Geometry check sheet. Reference: the model listing, model coordinates, mm. Round coordinates to 2 decimals unless told otherwise and drop trailing zeros. Order: outer loops, then holes, each group sorted by start corner. A loop starts at its lowest first (then second) coordinate and runs counter-clockwise, first axis right, second up. Notation, with made-up numbers: (41, 45) - (66, 45) arc R23 ccw to (66, 79) - close; hole circle Ø11 at (58, 89). An arc over 180 degrees is marked (long way). Write each question's results on one line, items separated by ' | '.
```python
from build123d import *

# Parameters (mm, degrees)
SKETCH1_W           = 313
SKETCH1_H           = 342
BOSS_EXTRUDE1_DEPTH = 6.35
SKETCH3_W           = 22
SKETCH3_H           = 155.14040353
SKETCH3_R           = 2.5
BOSS_EXTRUDE2_DEPTH = 6.35
SKETCH2_R           = 2.5
CUT_EXTRUDE1_DEPTH  = 7.35
SKETCH4_R           = 3.5
CUT_EXTRUDE2_DEPTH  = 7.35
SKETCH5_R           = 1.05
CUT_EXTRUDE3_DEPTH  = 7.35


with BuildPart() as part:
    # Sketch1 → Boss-Extrude1 (new body)
    with BuildSketch(Plane(origin=(0, 0, 0), x_dir=(1, 0, 0), z_dir=(0, 1, 0))):
        Rectangle(SKETCH1_W, SKETCH1_H)
    extrude(amount=-BOSS_EXTRUDE1_DEPTH)

    # Sketch3 → Boss-Extrude2 (add)
    with BuildSketch(Plane(origin=(0, 0, 0), x_dir=(1, 0, 0), z_dir=(0, 1, 0))):
        with Locations((167.5, 9)):
            Rectangle(SKETCH3_W, SKETCH3_H)
        with Locations((166.5, 9)):
            Circle(SKETCH3_R, mode=Mode.SUBTRACT)
        with Locations((166.5, -41.8)):
            Circle(SKETCH3_R, mode=Mode.SUBTRACT)
        with Locations((166.5, 59.8)):
            Circle(SKETCH3_R, mode=Mode.SUBTRACT)
    extrude(amount=-BOSS_EXTRUDE2_DEPTH)

    # Sketch2 → Cut-Extrude1 (cut, through all)
    with BuildSketch(Plane(origin=(0, 0, 0), x_dir=(1, 0, 0), z_dir=(0, 1, 0))):
        with Locations((0, -123)):
            Circle(SKETCH2_R)
        with Locations((-70, -123)):
            Circle(SKETCH2_R)
        with Locations((70, -123)):
            Circle(SKETCH2_R)
        with Locations((-70, 141)):
            Circle(SKETCH2_R)
        with Locations((0, 141)):
            Circle(SKETCH2_R)
        with Locations((70, 141)):
            Circle(SKETCH2_R)
    extrude(amount=-CUT_EXTRUDE1_DEPTH, mode=Mode.SUBTRACT)

    # Sketch4 → Cut-Extrude2 (cut, through all)
    with BuildSketch(Plane(origin=(0, 0, 0), x_dir=(1, 0, 0), z_dir=(0, 1, 0))):
        with Locations((133.64, -142.84)):
            Circle(SKETCH4_R)
        with Locations((108.24, -142.84)):
            Circle(SKETCH4_R)
    cut_extrude2 = extrude(amount=-CUT_EXTRUDE2_DEPTH, mode=Mode.SUBTRACT)

    # Mirror1: Cut-Extrude2 across plane
    add(cut_extrude2.mirror(Plane(origin=(0, 0, -9), x_dir=(1, 0, 0), z_dir=(0, 0, -1))), mode=Mode.SUBTRACT)

    # Sketch5 → Cut-Extrude3 (cut, through all)
    with BuildSketch(Plane(origin=(0, 0, 0), x_dir=(1, 0, 0), z_dir=(0, 1, 0))):
        with Locations((49.149172759, 77.943976756)):
            Circle(SKETCH5_R)
        with Locations((49.149172759, -67.056023244)):
            Circle(SKETCH5_R)
        with Locations((-45.850827241, 77.943976756)):
            Circle(SKETCH5_R)
        with Locations((-45.850827241, -67.056023244)):
            Circle(SKETCH5_R)
    extrude(amount=-CUT_EXTRUDE3_DEPTH, mode=Mode.SUBTRACT)


solid = part.part
```
(1) Material ranges on line 1 (Z direction, x = 0, y = -4); line 2 (Z direction, x = 2, y = -4.5); line 3 (X direction, y = -1.75, z = 123), recorded low to high.
Answers follow:
line 1: -171 to -143.5, -138.5 to 120.5, 125.5 to 171 | line 2: -171 to -142.5, -139.5 to 121.5, 124.5 to 171 | line 3: -156.5 to -72.5, -67.5 to -2.5, 2.5 to 67.5, 72.5 to 156.5
(2) Section check A-A (y = -3). Give the number of separate pieces and of enclosed holes in the cut face, then the cut area to 3 significant figures.
Answers follow:
separate pieces: 1 | enclosed holes: 17 | area: 110,000 mm²
(3) Section check B-B (z = -117.5). Record the cut outline in (x, y), then the cut area to 3 significant figures.
Answers follow:
outline: (-156.5, -6.35) - (156.5, -6.35) - (156.5, 0) - (-156.5, 0) - close | area: 1,990 mm²
